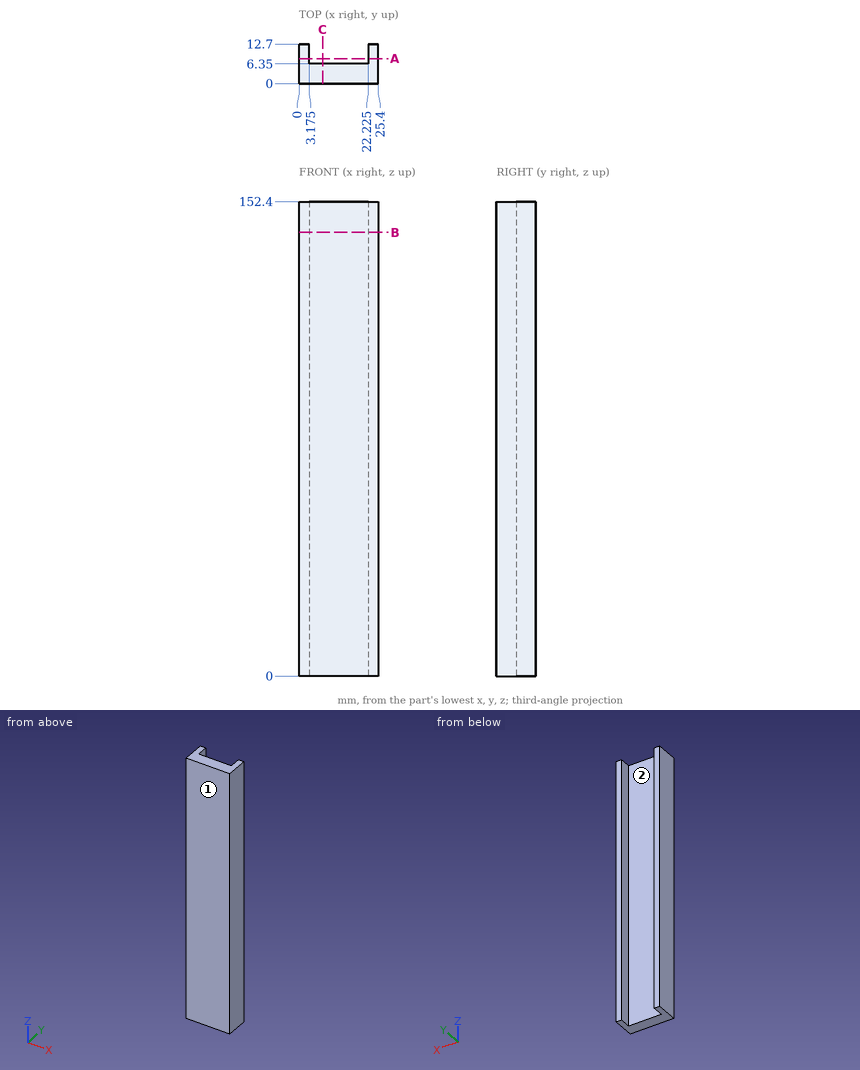
Geometry check sheet. Reference: drawing and pictorial views, mm from the part's lowest x, y, z. Coordinates: 2 decimals unless noted, no trailing zeros. Loops run counter-clockwise (first coordinate to the right, second up) from the corner with the lowest first, then second, coordinate; pieces in that order, holes last. Notation, with made-up numbers: (-31.5, -29) -> (7.5, -29) arc R19 ccw to (7.5, -10) -> close; hole circle Ø8 at (-34, -27.5). An arc over 180 degrees is marked (long way). Put each result on its own line as item: value.
1) Thickness scan on line 1 (X direction, y = 10.25, z = 30.5) (3 decimals); line 2 (Y direction, x = 4.25, z = 138.5). Record the ranges inside material, lowest first.
Result set:
line 1: x = 0 to 3.175, 22.225 to 25.4
line 2: y = 0 to 6.35
2) Cross-section at C-C on x = 7.5. Record the boundary of the cut face in (y, z).
Result set:
outline: (0, 0) -> (6.35, 0) -> (6.35, 152.4) -> (0, 152.4) -> close
3) Cross-section at A-A on y = 8. Record the boundary of the cut face in (x, z) (3 decimals).
Result set:
outline: (0, 0) -> (3.175, 0) -> (3.175, 152.4) -> (0, 152.4) -> close; (22.225, 0) -> (25.4, 0) -> (25.4, 152.4) -> (22.225, 152.4) -> close
4) Gauge pin test, flat ends, axial feed: pin 1 Ø6 at (x, y) = (3, 9) entering from -Z; pin 2 Ø5.5 at (x, z) = (17, 56.5) entering from +Y. Record the tip position at first contact, or that the pin passes through.
Result set:
pin 1: stops at z = 0
pin 2: stops at y = 6.35
5) Cross-section at B-B on z = 142.5. Record the boundary of the cut face in (x, y) (3 decimals), plus the area to 3 significant figures.
Result set:
outline: (0, 0) -> (25.4, 0) -> (25.4, 12.7) -> (22.225, 12.7) -> (22.225, 6.35) -> (3.175, 6.35) -> (3.175, 12.7) -> (0, 12.7) -> close
area: 202 mm^2
6) Release check for a two-part mould opening along X. For the marked faces 1 and 2 record: released by +X, released by -X, zero draft, split by the parting line, or undercut.
Result set:
face 1: zero draft
face 2: undercut
